Autodesk Inventor part; units mm, degrees
ref_plane "YZ Plane" through (0, 0, 0) normal (1, 0, 0) x (0, 1, 0)
ref_plane "XZ Plane" through (0, 0, 0) normal (0, 1, 0) x (-1, 0, 0)
ref_plane "XY Plane" through (0, 0, 0) normal (0, 0, 1) x (1, 0, 0)
sketch "Sketch1" plane through (0, 0, 0) normal (0, 1, 0) x (-1, 0, 0)
  line L0 (0, 0) -> (169, 0)
  line L1 (169, 0) -> (169, -20)
  line L2 (169, -20) -> (0, -20)
  line L3 (0, -20) -> (0, 0)
  dimension "d0" = 169
  dimension "d1" = 20
extrude "base" add sketch "Sketch1" along normal blind 2
sketch "Sketch2" plane through (0, 0, 0) normal (0, -1, 0) x (1, 0, 0)
  circle A0 centre (-160.5, -10) radius 2
  circle A1 centre (-8.5, -10) radius 2
  line L0 (-169, -20) -> (-169, 0) construction
  line L1 (-169, -10) -> (0, -10) construction
  line L2 (0, 0) -> (0, -20) construction
  dimension "d4" = 152
  dimension "d5" = 4
  dimension "d6" = 4
  dimension "d7" = 8.5
  dimension "d8" = 169
extrude "holes" cut sketch "Sketch2" against normal blind 2
sketch "Sketch3" plane through (0, 0, 0) normal (0, -1, 0) x (1, 0, 0)
  line L0 (0, 0) -> (0, -20) construction
  line L1 (0, -10) -> (-169, -10) construction
  line L2 (-169, -20) -> (-169, 0) construction
  circle A0 centre (-160.5, -10) radius 2 construction
  line L3 (-160.5, -10) -> (-160.5, 5.7595) construction
  circle A1 centre (-8.5, -10) radius 2 construction
  line L4 (-8.5, -10) -> (-8.5, 9.069) construction
  arc A2 (-143.25, -4) -> (-143.25, -16) centre (-143.25, -10) ccw
  line L5 (-143.25, -10) -> (-143.25, -16) construction
  line L6 (-143.25, -10) -> (-143.25, -4) construction
  line L7 (-143.25, -4) -> (-118.25, -4)
  line L8 (-143.25, -16) -> (-118.25, -16)
  arc A3 (-118.25, -16) -> (-118.25, -4) centre (-118.25, -10) ccw
  line L9 (-118.25, -10) -> (-118.25, -16) construction
  line L10 (-118.25, -10) -> (-118.25, -4) construction
  line L11 (-97, -4) -> (-72, -4)
  arc A4 (-97, -4) -> (-97, -16) centre (-97, -10) ccw
  line L12 (-97, -16) -> (-72, -16)
  arc A5 (-72, -16) -> (-72, -4) centre (-72, -10) ccw
  line L13 (-50.75, -4) -> (-25.75, -4)
  arc A6 (-50.75, -4) -> (-50.75, -16) centre (-50.75, -10) ccw
  line L14 (-50.75, -16) -> (-25.75, -16)
  arc A7 (-25.75, -16) -> (-25.75, -4) centre (-25.75, -10) ccw
  point P0 (-158.5, -10)
  point P1 (-10.5, -10)
  point P2 (-149.25, -10)
  dimension "d11" = 180
  dimension "d12" = 6
  dimension "d13" = 180
  dimension "d14" = 25
  dimension "d18" = 46.25
  dimension "d23" = 148
  dimension "d25" = 9.25
extrude "Extrusion3" cut sketch "Sketch3" against normal blind 10
equation "\"d6\" = d5"
equation "\"d7\" = -0.5 * d4 + 0.5 * d8"
equation "\"d18\" = 2 * d12 + d25 + d14"
equation "\"d24\" = -1.5 * d12 - 0.75 * d14 + 0.25 * d23"
properties part number "transverseClipStiffener" material "Steel"
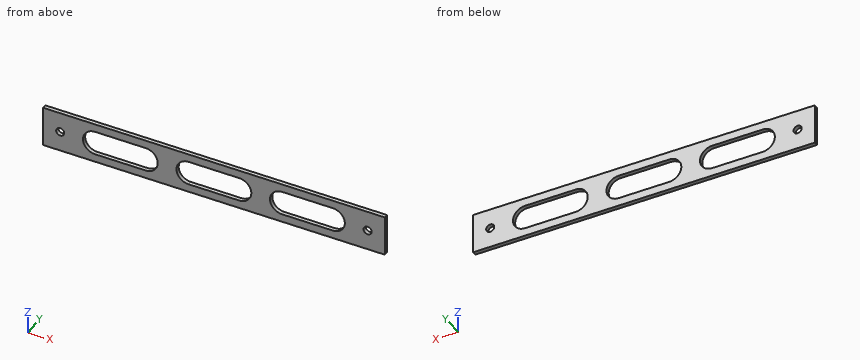
Check sheet for the modelled part. Datum: model origin and axes. Units: mm. Round coordinates to 2 decimals unless told otherwise and drop trailing zeros. Order: outer loops, then holes, each group sorted by start corner. A loop starts at its lowest first (then second) coordinate and runs counter-clockwise, first axis right, second up. Notation, with made-up numbers: (20.25, -29.5) -> (54.25, -29.5) arc R21 cw to (54.25, -17.5) -> close; hole circle Ø8 at (-12.75, 47.25). An arc over 180 degrees is marked (long way). One line per item, written item: value. Start each with the question number.
Q1. Thickness scan on line 1 (Z direction, x = -8.5, y = 1.25); line 2 (X direction, y = 1, z = -9); line 3 (X direction, y = 0.9, z = -14.5). Record the ranges inside material, lowest first.
Q2. Cross-section at A-A (x = -85.5). Record the boundary of the cut face in (y, z), and give its area (3 significant figures).
Q3. Cross-section at C-C (y = 1.2). Record the boundary of the cut face in (x, z).
Q4. Cross-section at B-B (z = -10). Record the boundary of the cut face in (x, y), and give its area (3 significant figures).
Q5. Cross-section at D-D (x = -160.5). Record the boundary of the cut face in (y, z).
Completed:
1. line 1: z = -20 to -12, -8 to 0
1. line 2: x = -169 to -162.23, -158.77 to -149.17, -112.33 to -102.92, -66.08 to -56.67, -19.83 to -10.23, -6.77 to 0
1. line 3: x = -169 to -147.22, -114.28 to -100.97, -68.03 to -54.72, -21.78 to 0
2. outline: (0, -20) -> (2, -20) -> (2, -16) -> (0, -16) -> close; (0, -4) -> (2, -4) -> (2, 0) -> (0, 0) -> close
2. area: 16.0 mm²
3. outline: (-169, -20) -> (0, -20) -> (0, 0) -> (-169, 0) -> close; hole circle Ø4 at (-160.5, -10); hole (-143.25, -16) -> (-118.25, -16) arc R6 ccw to (-118.25, -4) -> (-143.25, -4) arc R6 ccw to start; hole (-97, -16) -> (-72, -16) arc R6 ccw to (-72, -4) -> (-97, -4) arc R6 ccw to start; hole (-50.75, -16) -> (-25.75, -16) arc R6 ccw to (-25.75, -4) -> (-50.75, -4) arc R6 ccw to start; hole circle Ø4 at (-8.5, -10)
4. outline: (-169, 0) -> (-162.5, 0) -> (-162.5, 2) -> (-169, 2) -> close; (-158.5, 0) -> (-149.25, 0) -> (-149.25, 2) -> (-158.5, 2) -> close; (-112.25, 0) -> (-103, 0) -> (-103, 2) -> (-112.25, 2) -> close; (-66, 0) -> (-56.75, 0) -> (-56.75, 2) -> (-66, 2) -> close; (-19.75, 0) -> (-10.5, 0) -> (-10.5, 2) -> (-19.75, 2) -> close; (-6.5, 0) -> (0, 0) -> (0, 2) -> (-6.5, 2) -> close
4. area: 100 mm²
5. outline: (0, -20) -> (2, -20) -> (2, -12) -> (0, -12) -> close; (0, -8) -> (2, -8) -> (2, 0) -> (0, 0) -> close
